Could you check a few things on this model? Use its own coordinates, in mm. A direction names the side the tool comes from. Coordinates: 2 decimals unless noted, no trailing zeros. Loops run counter-clockwise (first coordinate to the right, second up) from the corner with the lowest first, then second, coordinate; pieces in that order, holes last.
1) Imagine slicing it at C-C on x = 70. Please give me the cut outline in (y, z).
2) Will these pins go through, and if not, where does the flat tip stop? P1, Ø1.5, axis at x = 45.5, y = 330, coming from the -Z side; P2, Ø22, axis at y = 289, z = -13, coming from the +X side.
3) For faces 1 (the face through (-7, 242, -20)), 2 (the face through (74, 242, 0)), which set-ups out of +Z, -Z, +X, -X, +Y, -Y let a thin tool reach every point of the face, with its end or its side?
4) Imagine slicing it at B-B on z = -8.5. Please give me the cut outline in (x, y), plus the area to 3 significant figures.
5) Imagine slicing it at A-A on y = 444.5. Please give me the cut outline in (x, z).
6) If I drill on line 1 along Z through (x, y) = (53.5, 25); line 2 along X through (y, z) = (340.5, 85); line 3 along X through (y, z) = (295, 86), over which ranges is the centre line in solid material (lowest first)?
```python
from build123d import *

# Parameters (mm, degrees)
PAD_DEPTH = 490
FILLET_R  = 18


with BuildPart() as part:
    # Sketch → Pad (new body)
    with BuildSketch(Plane.XZ):
        Polygon((0, 0), (150, 0), (150, 100), (0, 100), (-13, 100), (-13, -20), (0, -20), align=None)
    extrude(amount=-PAD_DEPTH)

    # Fillet
    fillet_edges = [part.edges().sort_by_distance(p)[0] for p in [
        (-13, 245, 100),
    ]]
    fillet(fillet_edges, radius=FILLET_R)


solid = part.part
```
Filled in:
1. outline: (0, 0) - (490, 0) - (490, 100) - (0, 100) - close
2. P1: stops at z = 0
2. P2: stops at x = 0
3. face 1: -Z, +X, -X, +Y, -Y
3. face 2: -Z, +X, +Y, -Y
4. outline: (-13, 0) - (0, 0) - (0, 490) - (-13, 490) - close
4. area: 6,370 mm2
5. outline: (-13, -20) - (0, -20) - (0, 0) - (150, 0) - (150, 100) - (5, 100) arc R18 ccw to (-13, 82) - close
6. line 1: z = 0 to 100
6. line 2: x = -12.75 to 150
6. line 3: x = -12.55 to 150
